Part model, mm, in its own coordinate system. Face numbers are marked on the shaded views. A direction names the side the tool comes from. Round coordinates to 2 decimals unless told otherwise and drop trailing zeros. Write each loop counter-clockwise with the first axis right and the second up, starting at its lowest first coordinate (ties: lowest second). Pieces come first, ordered by that corner, then holes.
1) Drill centre lines: L1, parallel to X at y = 0.2, z = 0; L2, parallel to X at y = 7.5, z = 0. Where is each one in solid material? Low to high.
2) Saw through at B-B on x = 0. Write the cut outline in (y, z).
3) Saw through at A-A on z = 0. Write the cut outline in (x, y).
4) Saw through at C-C on y = 4.75. Write the cut outline in (x, z), and give its area (3 significant figures).
5) Flat gauge pins, fed straight in: pin 1 (3 mm diameter, centred on y = 3, z = -29, fed in from +X); pin 2 (5 mm diameter, centred on x = 13, y = 2, fed in from +Z); pin 3 (1 mm diameter, centred on y = 2.5, z = -13, fed in from +X). Where does each tip first touch, or does it go through?
6) Pull direction Z, two halves, no side cores. Call the marked faces 1 and 2: +Z half, -Z half, draft (parallel to the pull), parting line (faces both ways), or undercut.
7) Which spindle directions (+Z, -Z, +X, -X, +Y, -Y) get a long thin tool onto all of the face, cutting with end or side? Do the marked faces 3 and 4. Say none if no direction does.
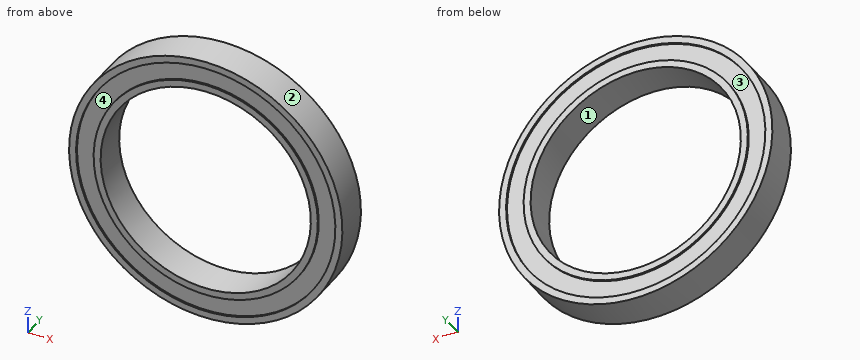
```python
from build123d import *

# Parameters (mm, degrees)
SKETCH1_R           = 39
SKETCH1_R_2         = 30
BOSS_EXTRUDE1_DEPTH = 10
SKETCH2_R           = 37
SKETCH2_R_2         = 32
CUT_EXTRUDE1_DEPTH  = 0.5
CUT_EXTRUDE2_START  = -0.5
SKETCH3_R           = 37
SKETCH3_R_2         = 32
CUT_EXTRUDE2_DEPTH  = 0.5


with BuildPart() as part:
    # Sketch1 → Boss-Extrude1 (new body)
    with BuildSketch(Plane(origin=(0, 0, 0), x_dir=(1, 0, 0), z_dir=(0, 1, 0))):
        with Locations(Location((0, 0, 0), (0, 0, 270))):
            Circle(SKETCH1_R)
        with Locations(Location((0, 0, 0), (0, 0, 270))):
            Circle(SKETCH1_R_2, mode=Mode.SUBTRACT)
    extrude(amount=BOSS_EXTRUDE1_DEPTH)

    # Sketch2 → Cut-Extrude1 (cut)
    with BuildSketch(Plane(origin=(0, 10, 0), x_dir=(1, 0, 0), z_dir=(0, 1, 0))):
        with Locations(Location((0, 0, 0), (0, 0, 270))):
            Circle(SKETCH2_R)
        with Locations(Location((0, 0, 0), (0, 0, 270))):
            Circle(SKETCH2_R_2, mode=Mode.SUBTRACT)
    extrude(amount=-CUT_EXTRUDE1_DEPTH, mode=Mode.SUBTRACT)

    # Sketch3 → Cut-Extrude2 (cut)
    with BuildSketch(Plane.XZ.offset(CUT_EXTRUDE2_START)):
        with Locations(Location((0, 0, 0), (0, 0, 90))):
            Circle(SKETCH3_R)
        with Locations(Location((0, 0, 0), (0, 0, 90))):
            Circle(SKETCH3_R_2, mode=Mode.SUBTRACT)
    extrude(amount=CUT_EXTRUDE2_DEPTH, mode=Mode.SUBTRACT)


solid = part.part
```
Completed:
1. L1: x = -39 to -37, -32 to -30, 30 to 32, 37 to 39
1. L2: x = -39 to -30, 30 to 39
2. outline: (0, -39) - (10, -39) - (10, -37) - (9.5, -37) - (9.5, -32) - (10, -32) - (10, -30) - (0, -30) - (0, -32) - (0.5, -32) - (0.5, -37) - (0, -37) - close; (0, 30) - (10, 30) - (10, 32) - (9.5, 32) - (9.5, 37) - (10, 37) - (10, 39) - (0, 39) - (0, 37) - (0.5, 37) - (0.5, 32) - (0, 32) - close
3. outline: (-39, 0) - (-37, 0) - (-37, 0.5) - (-32, 0.5) - (-32, 0) - (-30, 0) - (-30, 10) - (-32, 10) - (-32, 9.5) - (-37, 9.5) - (-37, 10) - (-39, 10) - close; (30, 0) - (32, 0) - (32, 0.5) - (37, 0.5) - (37, 0) - (39, 0) - (39, 10) - (37, 10) - (37, 9.5) - (32, 9.5) - (32, 10) - (30, 10) - close
4. outline: circle Ø78 at (0, 0); hole circle Ø60 at (0, 0)
4. area: 1,950 mm2
5. pin 1: stops at x = 27.65
5. pin 2: stops at z = 37.56
5. pin 3: stops at x = 36.94
6. face 1: undercut
6. face 2: parting line
7. face 3: +Y
7. face 4: -Y
